Check sheet for the modelled part. Datum: model origin and axes. Units: mm. Coordinates: 2 decimals unless noted, no trailing zeros. Loops run counter-clockwise (first coordinate to the right, second up) from the corner with the lowest first, then second, coordinate; pieces in that order, holes last. Notation, with made-up numbers: M 81,-30.75 L 133,-30.75 A28 ccw 133,-5.75 Z; hole C -26,-9.5 d11. An arc over 180 degrees is marked long. Return JSON: item names as keys, results as strings.
from build123d import *

# Parameters (mm, degrees)
CROQUIS1_W              = 245
CROQUIS1_H              = 215.984697531
CROQUIS1_R              = 6.1
SALIENTE_EXTRUIR1_DEPTH = 2
CROQUIS2_W              = 40
CROQUIS2_H              = 30
SALIENTE_EXTRUIR2_DEPTH = 4
REDONDEO1_R             = 2


with BuildPart() as part:
    # Croquis1 → Saliente-Extruir1 (new body)
    with BuildSketch(Plane.XY):
        with Locations((0, -173.507651235)):
            Rectangle(CROQUIS1_W, CROQUIS1_H)
        with Locations((-108.504553774, -269.266081741)):
            Circle(CROQUIS1_R, mode=Mode.SUBTRACT)
        with Locations((108.504553774, -269.266081741)):
            Circle(CROQUIS1_R, mode=Mode.SUBTRACT)
        with Locations((108.504553774, -77.749220728)):
            Circle(CROQUIS1_R, mode=Mode.SUBTRACT)
        with Locations((-108.504553774, -77.749220728)):
            Circle(CROQUIS1_R, mode=Mode.SUBTRACT)
    extrude(amount=SALIENTE_EXTRUIR1_DEPTH)

    # Croquis2 → Saliente-Extruir2 (add)
    with BuildSketch(Plane(origin=(0, 0, 0), x_dir=(-1, 0, 0), z_dir=(0, 0, -1))):
        with Locations((0, -80.515302469)):
            Rectangle(CROQUIS2_W, CROQUIS2_H)
    extrude(amount=SALIENTE_EXTRUIR2_DEPTH)

    # Redondeo1
    redondeo1_edges = [part.edges().sort_by_distance(p)[0] for p in [
        (-20, -80.515302469, -4),
        (-20, -80.515302469, 0),
        (0, -95.515302469, 0),
        (20, -80.515302469, 0),
        (0, -95.515302469, -4),
        (20, -80.515302469, -4),
    ]]
    fillet(redondeo1_edges, radius=REDONDEO1_R - 0.0001)  # a hair under: the kernel refuses the full size


solid = part.part
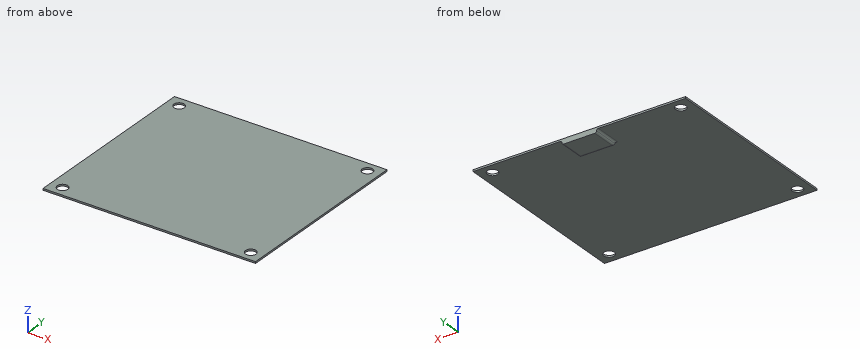
1) Go/stop test with flat-tipped pins: pin 1 Ø19.5 at (x, y) = (108.5, -77.75) entering from -Z; pin 2 Ø1 at (y, z) = (-90.5, -1) entering from +X. Record where each tip stops, or that it passes through.
Answers:
{"pin 1": "z = 0", "pin 2": "x = 20.68"}
2) Section check B-B on y = -206.5. Record the cut outline in (x, z), then the cut area to 3 significant figures.
Answers:
{"outline": "M -122.5,0 L 122.5,0 L 122.5,2 L -122.5,2 Z", "area": "490 mm²"}
3) Section check A-A on x = -85. Record the cut outline in (y, z), then the cut area to 3 significant figures.
Answers:
{"outline": "M -281.5,0 L -65.52,0 L -65.52,2 L -281.5,2 Z", "area": "432 mm²"}
4) Scan lines: line 1 along Z through (x, y) = (-31, -249.5); line 2 along X through (y, z) = (-73.5, -2); line 3 along X through (y, z) = (-82.5, -2.55). Record each from-to range of solid material in increasing order. Write a range as [from, to].
Answers:
{"line 1": "[0, 2]", "line 2": "[-20, 20]", "line 3": "[-19.92, 19.92]"}
